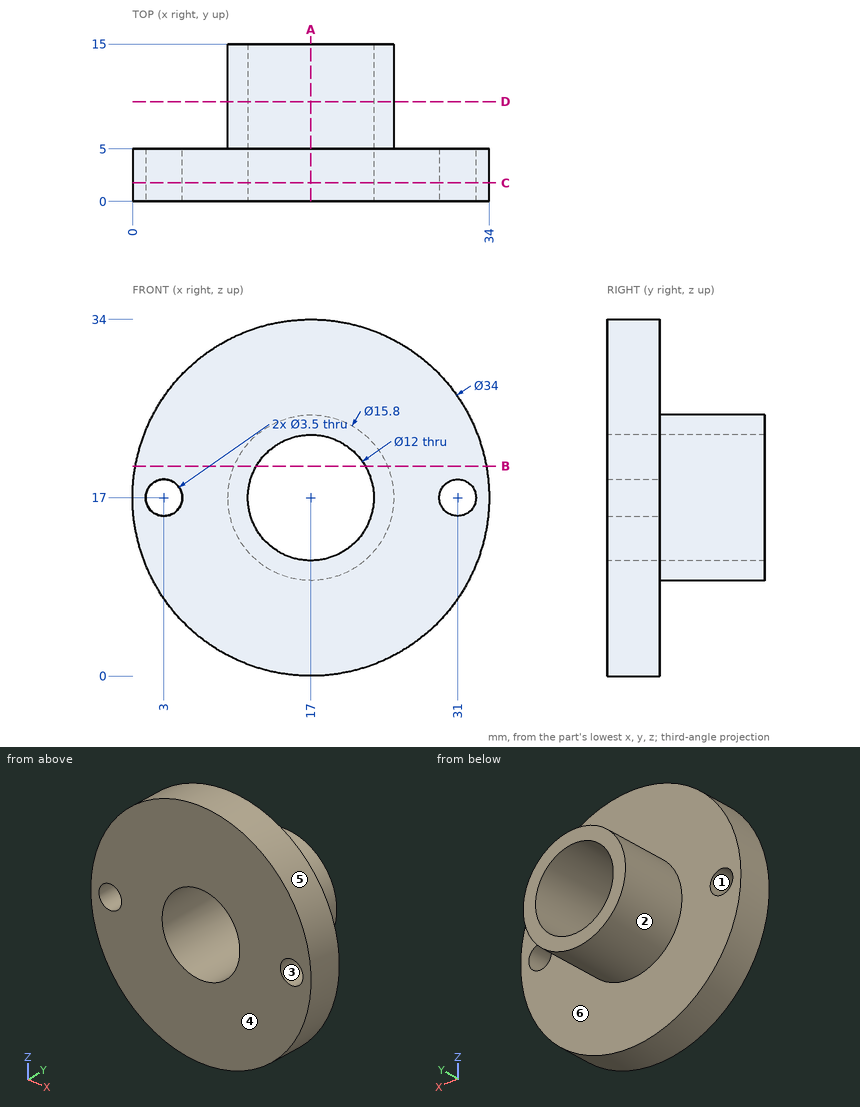
Study the drawing (mm; zero at the part's minimum x, y, z) and answer. A direction names the side the tool comes from. Coordinates: 2 decimals unless noted, no trailing zeros. Write each loop counter-clockwise with the first axis right and the second up, starting at its lowest first coordinate (ties: lowest second). Pieces come first, ordered by that corner, then holes. Notation, with made-up numbers: (29.5, 69.5) - (53.5, 69.5) arc R29 ccw to (53.5, 96.5) - close; hole circle Ø7 at (51, 12). An arc over 180 degrees is marked (long way). Return JSON: item names as keys, results as strings. Group by question number.
1. A cutting plane is placed at A-A, the plane x = 17. Determine the outline of the cut face in (y, z).
2. Determine the mould class of the marked faces 1, 2, 3 and 4 for opening direction Z: released by +Z, released by -Z, zero draft, split by the parting line, or undercut.
3. Given pin 1 (1.5 mm diameter, centred on x = 23, y = 3.5, fed in from -Z); pin 2 (2 mm diameter, centred on x = 8, y = 7.5, fed in from +Z); pin 3 (2 mm diameter, centred on x = 21.5, y = 1.5, fed in from +Z); pin 4 (5.5 mm diameter, centred on x = 3, z = 17, fed in from +Y), each flat-ended and moving along its own axis, determine where each tip first touches the part or whether it passes through.
4. A cutting plane is placed at B-B, the plane z = 20. Determine the outline of the cut face in (x, y), plus the area to 3 significant figures.
5. A cutting plane is placed at D-D, the plane y = 9.5. Determine the outline of the cut face in (x, z), plus the area to 3 significant figures.
6. A cutting plane is placed at C-C, the plane y = 1.75. Determine the outline of the cut face in (x, z).
7. Which of the six approach directions +Z, -Z, +X, -X, +Y, -Y give full straight-line access (tool end or side, diameter ignored) to the marked faces 5 and 6?
8. Straight lines are drawn through the part: L1, parallel to Z at x = 17, y = 10.75; L2, parallel to Y at x = 15.5, z = 25; L3, parallel to Z at x = 13.5, y = 10.25. For each, find the intervals that lie inside material, in ascending order.
Ans:
{
 "1": {"outline": "(0, 0) - (5, 0) - (5, 9.1) - (15, 9.1) - (15, 11) - (0, 11) - close; (0, 23) - (15, 23) - (15, 24.9) - (5, 24.9) - (5, 34) - (0, 34) - close"},
 "2": {"face 1": "undercut", "face 2": "split by the parting line", "face 3": "undercut", "face 4": "zero draft"},
 "3": {"pin 1": "z = 0.83", "pin 2": "through", "pin 3": "z = 33.64", "pin 4": "y = 5"},
 "4": {"outline": "(0.27, 0) - (11.8, 0) - (11.8, 15) - (9.69, 15) - (9.69, 5) - (0.27, 5) - close; (22.2, 0) - (33.73, 0) - (33.73, 5) - (24.31, 5) - (24.31, 15) - (22.2, 15) - close", "area": "158 mm²"},
 "5": {"outline": "circle Ø15.8 at (17, 17); hole circle Ø12 at (17, 17)", "area": "83.0 mm²"},
 "6": {"outline": "circle Ø34 at (17, 17); hole circle Ø3.5 at (3, 17); hole circle Ø12 at (17, 17); hole circle Ø3.5 at (31, 17)"},
 "7": {"face 5": "+Y, -Y", "face 6": "+Y"},
 "8": {"L1": "9.1 to 11, 23 to 24.9", "L2": "0 to 5", "L3": "9.92 to 12.13, 21.87 to 24.08"}
}
